Source: CAD feature listing. Evaluate the final solid. Frame: model axes, mm. Face numbers are marked on the shaded views. A direction names the side the tool comes from. Give positions to 0.01 mm unless a question says otherwise; leave off trailing zeros. Order: outer loops, then holes, each group sorted by start corner. A loop starts at its lowest first (then second) coordinate and runs counter-clockwise, first axis right, second up.
from build123d import *

# Parameters (mm, degrees)
SKETCH1_R           = 1.1
SKETCH1_W           = 8.5
SKETCH1_H           = 8.5
BOSS_EXTRUDE1_DEPTH = 3.175


with BuildPart() as part:
    # Sketch1 → Boss-Extrude1 (new body)
    with BuildSketch(Plane.XY):
        with BuildLine():
            Line((-10.705332644, 7.071510672), (10.294667356, 7.071510672))
            ThreePointArc((10.294667356, 7.071510672), (11.708880919, 6.485724235), (12.294667356, 5.071510672))
            Line((12.294667356, 5.071510672), (12.294667356, -14.928489328))
            ThreePointArc((12.294667356, -14.928489328), (11.708880919, -16.34270289), (10.294667356, -16.928489328))
            Line((10.294667356, -16.928489328), (-10.705332644, -16.928489328))
            ThreePointArc((-10.705332644, -16.928489328), (-12.119546206, -16.34270289), (-12.705332644, -14.928489328))
            Line((-12.705332644, -14.928489328), (-12.705332644, 5.071510672))
            ThreePointArc((-12.705332644, 5.071510672), (-12.119546206, 6.485724235), (-10.705332644, 7.071510672))
        make_face()
        with Locations((-10.705332644, -14.928489328)):
            Circle(SKETCH1_R, mode=Mode.SUBTRACT)
        with Locations((-10.705332644, -2.390489328)):
            Circle(SKETCH1_R, mode=Mode.SUBTRACT)
        with Locations((10.294667356, -2.390489328)):
            Circle(SKETCH1_R, mode=Mode.SUBTRACT)
        with Locations((10.294667356, -14.928489328)):
            Circle(SKETCH1_R, mode=Mode.SUBTRACT)
        with Locations((-0.205332644, -2.678489328)):
            Rectangle(SKETCH1_W, SKETCH1_H, mode=Mode.SUBTRACT)
    extrude(amount=-BOSS_EXTRUDE1_DEPTH)


solid = part.part
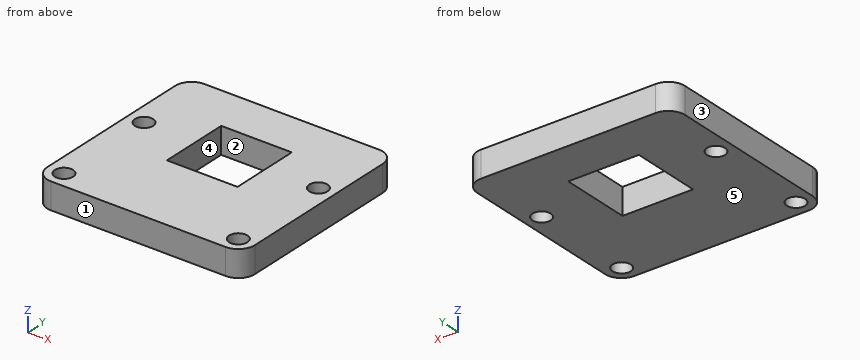
(1) Access query for the marked faces 4 and 5. Directions: +Z, -Z, +X, -X, +Y, -Y. A direction counts if a zero-diameter tool reaches every point of the face in a straight line with its end or side. Return the directions, or none.
(2) Section C-C, the plane z = -0.8. Return loops of the section in (x, y).
(3) Draft query along Y for the marked faces 1, 2 and 3. Return one class per face: +Y half, -Y half, draft (parallel to the pull), parting line (faces both ways), or undercut.
(4) Section B-B, the plane y = -4.5. Return loops of the section in (x, z) (3 decimals), plus the area to 3 significant figures.
(5) Section D-D, the plane y = -14.5. Return loops of the section in (x, z) (3 decimals), plus the area to 3 significant figures.
(6) Line query: line 1 along Y through (x, z) = (0.25, -1.1); line 2 along X through (y, z) = (-3.75, -1.35); line 3 along X through (y, z) = (-1.5, -0.6). Output: solid intervals per line, ascending.
(7) Section A-A, the plane x = 1.25. Return loops of the section in (y, z) (3 decimals), plus the area to 3 significant figures.
(8) Pin query (flat end, axial travel): pin 1 Ø2 at (x, y) = (10.29, -2.39) entering from -Z. Return the tip coordinate at first contact, or that it passes through.
Checks:
1. face 4: +Z, -Z
1. face 5: -Z, +X, -X, +Y, -Y
2. outline: (-12.71, -14.93) arc R2 ccw to (-10.71, -16.93) - (10.29, -16.93) arc R2 ccw to (12.29, -14.93) - (12.29, 5.07) arc R2 ccw to (10.29, 7.07) - (-10.71, 7.07) arc R2 ccw to (-12.71, 5.07) - close; hole circle Ø2.2 at (-10.71, -14.93); hole circle Ø2.2 at (-10.71, -2.39); hole (-4.46, -6.93) - (4.04, -6.93) - (4.04, 1.57) - (-4.46, 1.57) - close; hole circle Ø2.2 at (10.29, -14.93); hole circle Ø2.2 at (10.29, -2.39)
3. face 1: -Y half
3. face 2: undercut
3. face 3: draft
4. outline: (-12.705, -3.175) - (-4.455, -3.175) - (-4.455, 0) - (-12.705, 0) - close; (4.045, -3.175) - (12.295, -3.175) - (12.295, 0) - (4.045, 0) - close
4. area: 52.4 mm2
5. outline: (-12.705, -3.175) - (-11.718, -3.175) - (-11.718, 0) - (-12.705, 0) - close; (-9.692, -3.175) - (9.282, -3.175) - (9.282, 0) - (-9.692, 0) - close; (11.308, -3.175) - (12.295, -3.175) - (12.295, 0) - (11.308, 0) - close
5. area: 66.5 mm2
6. line 1: y = -16.93 to -6.93, 1.57 to 7.07
6. line 2: x = -12.71 to -4.46, 4.04 to 12.29
6. line 3: x = -12.71 to -11.35, -10.06 to -4.46, 4.04 to 9.65, 10.94 to 12.29
7. outline: (-16.928, -3.175) - (-6.928, -3.175) - (-6.928, 0) - (-16.928, 0) - close; (1.572, -3.175) - (7.072, -3.175) - (7.072, 0) - (1.572, 0) - close
7. area: 49.2 mm2
8. pin 1: passes through
